Geometry check sheet. Reference: the model listing, model coordinates, mm. A direction names the side the tool comes from. Round coordinates to 2 decimals unless told otherwise and drop trailing zeros. Loops run counter-clockwise (first coordinate to the right, second up) from the corner with the lowest first, then second, coordinate; pieces in that order, holes last. Notation, with made-up numbers: (80, 6) - (121, 6) arc R26 cw to (121, 37) - close; hole circle Ø8 at (44.25, 57.5). An arc over 180 degrees is marked (long way). Answer in a Markdown table with one row per item. Add a question column.
Autodesk Inventor part; units mm, degrees
ref_plane "YZ Plane" through (0, 0, 0) normal (1, 0, 0) x (0, 1, 0)
ref_plane "XZ Plane" through (0, 0, 0) normal (0, 1, 0) x (-1, 0, 0)
ref_plane "XY Plane" through (0, 0, 0) normal (0, 0, 1) x (1, 0, 0)
sketch "Sketch1" plane through (0, 0, 0) normal (1, 0, 0) x (0, 1, 0)
  line L0 (10, 0) -> (58, 0)
  line L1 (78, -10) -> (78, -21)
  line L2 (78, -21) -> (78, -10)
  line L3 (78, -21) -> (78, -10)
  line L4 (78, -10) -> (78, -21)
  line L5 (58, 0) -> (10, 0)
  line L6 (58, 0) -> (10, 0)
  line L7 (78, -21) -> (78, -6)
  line L8 (78, -6) -> (58, 0)
  line L9 (78, -21) -> (76, -21)
  line L10 (76, -21) -> (76, -8)
  line L11 (10, -8) -> (76, -8)
  line L12 (10, -8) -> (10, 0)
  point P0 (0, 0)
  dimension "d6" = 15
  dimension "d9" = 2
extrude "Extrusion1" add sketch "Sketch1" along normal blind 779.45
properties part number "Blackside" material "Steel"
Q1. Scan lines: line 1 (Z direction, x = 32.5, y = 40); line 2 (Y direction, x = 166, z = -17.25); line 3 (Z direction, x = 129.5, y = 58.5). Record each from-to range of solid material in increasing order. Write a range as from..to.
Q2. Cross-section at C-C, the plane z = -17.5. Enter the section's corners in (x, y).
Q3. Cross-section at A-A, the plane x = 619. Enter the section's corners in (y, z), plus the area to 3 significant figures.
Q4. Release check for a two-part mould opening along Y. For faces 3 (the flat face through (384, 78, -13)), 4 (the flat face through (384, 76, -15)), 5 (the flat face through (0, 44, -5)) record: +Y half, -Y half, draft (parallel to the pull), parting line (faces both ways), or undercut.
Q5. Depth check by flat-ended pin: P1, Ø8, axis at x = 556, y = 68, coming from the -Z side; P2, Ø4, axis at x = 350, z = -17, coming from the -Y side; P3, Ø1.5, axis at y = 23, z = -9.5, coming from the -X side. Enter the tip coordinate at first touch or a pass-through.
Q6. Cross-section at B-B, the plane y = 65. Enter the section's corners in (x, z).
Q7. Set-up check for faces 1 (the flat face through (384, 68, -3)), 2 (the flat face through (384, 43, -8)): record each of +Z, -Z, +X, -X, +Y, -Y from which the full face is reachable in a straight line by a thin tool's end or side.
Check sheet entries:
| question | item | result |
|---|---|---|
| 1 | line 1 | -8..0 |
| 1 | line 2 | 76..78 |
| 1 | line 3 | -8..-0.15 |
| 2 | outline | (0, 76) - (779.45, 76) - (779.45, 78) - (0, 78) - close |
| 3 | outline | (10, -8) - (76, -8) - (76, -21) - (78, -21) - (78, -6) - (58, 0) - (10, 0) - close |
| 3 | area | 510 mm² |
| 4 | face 3 | +Y half |
| 4 | face 4 | -Y half |
| 4 | face 5 | draft |
| 5 | P1 | z = -8 |
| 5 | P2 | y = 76 |
| 5 | P3 | through |
| 6 | outline | (0, -8) - (779.45, -8) - (779.45, -2.1) - (0, -2.1) - close |
| 7 | face 1 | +Z, +X, -X, +Y |
| 7 | face 2 | -Z, +X, -X, -Y |
